Source: CAD feature listing. Evaluate the final solid. Frame: model axes, mm. Face numbers are marked on the shaded views. A direction names the side the tool comes from. Coordinates: 2 decimals unless noted, no trailing zeros. Order: outer loops, then holes, each group sorted by start corner. A loop starts at its lowest first (then second) coordinate and runs counter-clockwise, first axis right, second up.
Item 1: Mould query, pull axis X, two halves, no side actions, for the marked faces 4, 5 and 6. Classes: released by +X, released by -X, zero draft, split by the parting line, or undercut.
Item 2: Ray query, line 1 (Y direction, x = 60, z = -4.5); line 2 (X direction, y = 140, z = 34.5); line 3 (Z direction, x = 154.5, y = 190). Return the intervals inside material, ascending.
Item 3: Section C-C on y = 42.5. Return the cut outline in (x, z), then the cut area to 3 significant figures.
Item 4: Contact query for flat-ended pins moving along their axis: P1, Ø5, axis at y = 59.5, z = -10, coming from the +X side; P2, Ø3, axis at x = -104, y = 182, coming from the -Z side; P3, Ø4, axis at y = 197, z = 27.5, coming from the -X side. Output: stop coordinate, or through.
Item 5: Section D-D on x = -85. Return the cut outline in (y, z).
Item 6: Section A-A on z = 0. Return the cut outline in (x, y), then the cut area to 3 significant figures.
Item 7: Section B-B on x = 55. Return the cut outline in (y, z), then the cut area to 3 significant figures.
Item 8: Reachability of the marked faces 1, 2 and 3 from +Z, -Z, +X, -X, +Y, -Y: full face, straight path, thin tool, end or side. Return the list, or none.
from build123d import *

# Parameters (mm, degrees)
BOSS_EXTRUDE1_DEPTH      = 76.2
BOSS_EXTRUDE6_DEPTH      = 203.2
BOSS_EXTRUDE6_DEPTH_BACK = 152.4
CUT_EXTRUDE1_DEPTH       = 397.760683536
SKETCH9_W                = 152.4
SKETCH9_H                = 70.280514467
CUT_EXTRUDE2_DEPTH       = 475.511158984
SKETCH10_R               = 12.7
BOSS_EXTRUDE7_DEPTH      = 2.54
SKETCH11_W               = 58.732266579
SKETCH11_H               = 35.638828091
CUT_EXTRUDE3_DEPTH       = 316.168697926


with BuildPart() as part:
    # Sketch1 → Boss-Extrude1 (new, symmetric)
    with BuildSketch(Plane.XY):
        Polygon((0, 0), (50.8, 0), (25.4, 35.638828091), align=None)
    extrude(amount=BOSS_EXTRUDE1_DEPTH, both=True)

    # Sketch7 → Boss-Extrude6 (add, two sides: drawn at the far end of the back side and taken through both)
    with BuildSketch(Plane(origin=(0, 0, 0), x_dir=(0, 0, -1), z_dir=(1, 0, 0)).offset(-BOSS_EXTRUDE6_DEPTH_BACK)):
        Polygon((76.2, 234.519485533), (76.2, 304.8), (-76.2, 304.8), (-76.2, 234.519485533), (-5.035820147, 15.498660762), (5.035820147, 15.498660762), align=None)
    extrude(amount=BOSS_EXTRUDE6_DEPTH + BOSS_EXTRUDE6_DEPTH_BACK)

    # Sketch8 → Cut-Extrude1 (cut, through all)
    with BuildSketch(Plane.XY.offset(76.2)):
        Polygon((-145.479084616, 234.519485533), (-152.4, 234.519485533), (-152.4, 15.498660762), (-9.614258599, 15.498660762), align=None)
        Polygon((60.413322139, 15.498660762), (196.264914484, 234.519485533), (203.2, 234.519485533), (203.2, 15.498660762), align=None)
    extrude(amount=-CUT_EXTRUDE1_DEPTH, mode=Mode.SUBTRACT)

    # Sketch9 → Cut-Extrude2 (cut, through all)
    with BuildSketch(Plane(origin=(203.2, 0, 0), x_dir=(0, 0, -1), z_dir=(1, 0, 0))):
        with Locations((0, 269.659742767)):
            Rectangle(SKETCH9_W, SKETCH9_H)
    extrude(amount=-CUT_EXTRUDE2_DEPTH, mode=Mode.SUBTRACT)

    # Sketch10 → Boss-Extrude7 (add)
    with BuildSketch(Plane(origin=(0, 0, 0), x_dir=(-1, 0, 0), z_dir=(0, -1, 0))):
        with Locations(Location((0, 0, 0), (0, 0, 90))):
            Circle(SKETCH10_R)
        with Locations(Location((-50.8, 0, 0), (0, 0, 90))):
            Circle(SKETCH10_R)
    extrude(amount=BOSS_EXTRUDE7_DEPTH)

    # Sketch11 → Cut-Extrude3 (cut, through all)
    with BuildSketch(Plane(origin=(50.8, 0, 0), x_dir=(0, 0, -1), z_dir=(1, 0, 0))):
        with Locations((-46.833866711, 17.819414046)):
            Rectangle(SKETCH11_W, SKETCH11_H)
        with Locations((46.833866711, 17.819414046)):
            Rectangle(SKETCH11_W, SKETCH11_H)
    extrude(amount=-CUT_EXTRUDE3_DEPTH, mode=Mode.SUBTRACT)


solid = part.part
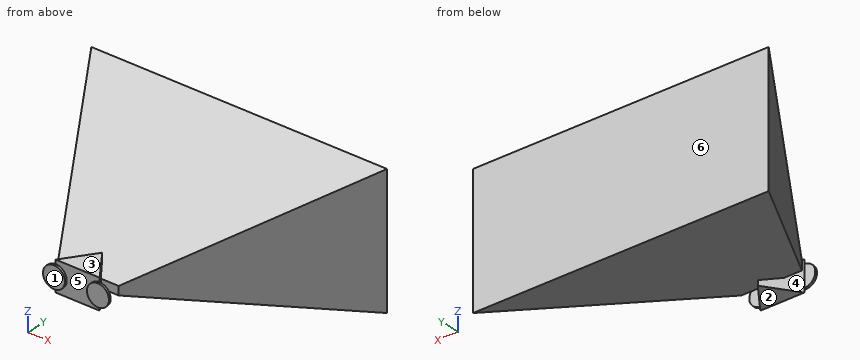
Answer list:
1. face 4: released by -X
1. face 5: undercut
1. face 6: zero draft
2. line 1: y = -2.54 to 0, 15.5 to 234.52
2. line 2: x = -86.85 to 137.64
2. line 3: z = -61.73 to 61.73
3. outline: (-26.36, -13.81) - (77.16, -13.81) - (77.16, 13.81) - (-26.36, 13.81) - close
3. area: 2,860 mm2
4. P1: stops at x = 89.26
4. P2: stops at z = -59.62
4. P3: stops at x = -123.45
5. outline: (137.02, -44.52) - (234.52, -76.2) - (234.52, 76.2) - (137.02, 44.52) - close
6. outline: (-145.48, 234.52) - (-9.61, 15.5) - (11.05, 15.5) - (0, 0) - (-12.7, 0) - (-12.7, -2.54) - (12.7, -2.54) - (12.7, 0) - (38.1, 0) - (38.1, -2.54) - (63.5, -2.54) - (63.5, 0) - (50.8, 0) - (39.75, 15.5) - (60.41, 15.5) - (196.26, 234.52) - close
6. area: 45,800 mm2
7. outline: (-2.54, -11.99) - (0, -11.99) - (0, 11.99) - (-2.54, 11.99) - close; (15.5, -5.04) - (234.52, -76.2) - (234.52, 76.2) - (15.5, 5.04) - close
7. area: 17,900 mm2
8. face 1: +Z, -Z, +X, -X, -Y
8. face 2: -Z, +X, -X, -Y
8. face 3: +Z, +X, -X, -Y
